from build123d import *

# Parameters (mm, degrees)
F0_W     = 150
F0_H     = 35
F1_DEPTH = 60
F2_W     = 10
F2_H     = 30
F3_DEPTH = 150
F4_W     = 75
F4_H     = 20
F5_DEPTH = 35.001
F6_R     = 10
F8_DEPTH = 35.001


with BuildPart() as f1:
    # F0 (on Top) → F1 (new body)
    with BuildSketch(Plane.XY):
        Rectangle(F0_W, F0_H)
    extrude(amount=F1_DEPTH)

    # F2 (on face) → F3 (cut)
    with BuildSketch(Plane.YZ.offset(75)):
        with Locations((0, 45)):
            Rectangle(F2_W, F2_H)
    extrude(amount=-F3_DEPTH, mode=Mode.SUBTRACT)

    # F4 (on face) → F5 (cut, through all)
    with BuildSketch(Plane.XZ.offset(17.5)):
        with Locations((-37.5, 10)):
            Rectangle(F4_W, F4_H)
    extrude(amount=-F5_DEPTH, mode=Mode.SUBTRACT)

    # F6
    f6_edges = [f1.edges().sort_by_distance(p)[0] for p in [
        (0, 0, 20),
    ]]
    fillet(f6_edges, radius=F6_R)

    # F7 (on face) → F8 (cut, through all)
    with BuildSketch(Plane.XZ.offset(17.5)):
        Polygon((15, 60), (-75, 60), (-75, 50), (0, 50), align=None)
    extrude(amount=-F8_DEPTH, mode=Mode.SUBTRACT)


solid = f1.part
Read the model definition and answer for the solid it produces. Units are mm, in the model's axes. A direction names the side the tool comes from. Give positions to 0.01 mm unless a question says otherwise; leave off trailing zeros. Write each loop counter-clockwise with the first axis right and the second up, starting at its lowest first coordinate (ties: lowest second). Pieces come first, ordered by that corner, then holes. Notation, with made-up numbers: M 70.25,-38 L 128.25,-38 A14 ccw 128.25,-11 Z; hole C 28.25,86 d5. An arc over 180 degrees is marked long. One line per item, written item: value. Start each with the question number.
(1) Find section C-C (y = -14.5). Determine the outline of the cut face in (x, z), plus the area to 3 significant figures.
(2) Determine the mould class of faces 1 (the flat face through (16, -17.5, 30)), 2 (the flat face through (1, 5, 41)), 3 (the flat face through (-38, 11, 50)), 4 (the flat face through (1, -5, 41)) for opening direction Y: pulls with the +Y half, pulls with the -Y half, needs draft (parallel to the pull), parting line crosses it, or undercut.
(3) Find section A-A (z = 43). Determine the outline of the cut face in (x, y), plus the area to 3 significant figures.
(4) Find the intervals of material crossed by line 1 (Y direction, x = 15, z = 52.5); line 2 (Z direction, x = 44, y = -3.5); line 3 (Z direction, x = -11.5, y = -8), in increasing order.
(5) Find section B-B (x = -34). Determine the outline of the cut face in (y, z), plus the area to 3 significant figures.
(6) Flat-ended cylindrical pins translate along their axes: pin 1 Ø1.5 at (x, y) = (-42.5, -12) entering from -Z; pin 2 Ø3 at (x, y) = (15, -1.5) entering from +Z; pin 3 Ø12 at (y, z) = (-3.5, 53) entering from +X; pin 4 Ø14 at (x, y) = (-52.5, 12) entering from +Z. Find the tip coordinate at first contact, or state that the pin passes through.
(7) A tool of negligible diameter and unlimited length cuts with its end or side. For faces 5 (the flat face through (-38, -11, 50)), 6 (the flat face through (-43, 0, 20)), 7 (the flat face through (1, 0, 30)), 8 (the flat face through (-75, 0, 28)), 9 (the flat face through (45, 11, 60)), from which of +Z, -Z, +X, -X, +Y, -Y can it reach the whole face along a straight path? Write none if from no direction.
(8) Find section D-D (y = -1.5). Determine the outline of the cut face in (x, z), plus the area to 3 significant figures.
Results below:
1. outline: M -75,20 L -10,20 A10 cw 0,10 L 0,0 L 75,0 L 75,60 L 15,60 L 0,50 L -75,50 Z
1. area: 6,700 mm^2
2. face 1: pulls with the -Y half
2. face 2: undercut
2. face 3: needs draft
2. face 4: undercut
3. outline: M -75,-17.5 L 75,-17.5 L 75,-5 L -75,-5 Z; M -75,5 L 75,5 L 75,17.5 L -75,17.5 Z
3. area: 3,750 mm^2
4. line 1: y = -17.5 to -5, 5 to 17.5
4. line 2: z = 0 to 30
4. line 3: z = 20 to 50
5. outline: M -17.5,20 L 17.5,20 L 17.5,50 L 5,50 L 5,30 L -5,30 L -5,50 L -17.5,50 Z
5. area: 850 mm^2
6. pin 1: stops at z = 20
6. pin 2: stops at z = 30
6. pin 3: stops at x = 75
6. pin 4: stops at z = 50
7. face 5: +Z, -X, +Y, -Y
7. face 6: -Z, -X, +Y, -Y
7. face 7: +Z, +X, -X
7. face 8: +Z, -Z, -X, +Y, -Y
7. face 9: +Z, +X, -X, +Y, -Y
8. outline: M -75,20 L -10,20 A10 cw 0,10 L 0,0 L 75,0 L 75,30 L -75,30 Z
8. area: 3,020 mm^2
